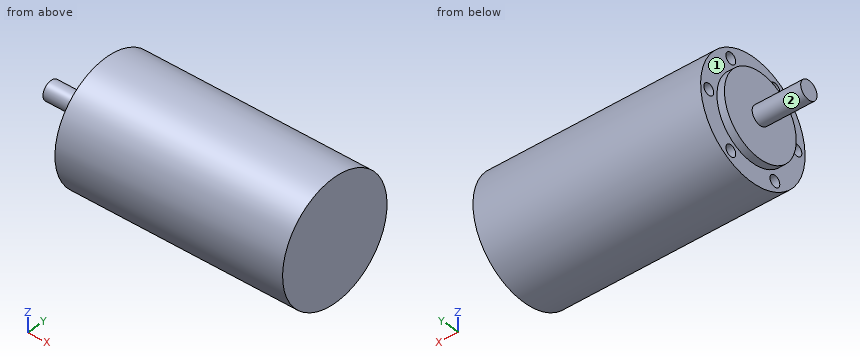
from build123d import *

# Parameters (mm, degrees)
SKETCH1_R           = 16
BOSS_EXTRUDE1_DEPTH = 61
SKETCH2_R           = 11
BOSS_EXTRUDE2_DEPTH = 2
SKETCH3_R           = 1.5
CUT_EXTRUDE1_DEPTH  = 4
SKETCH4_R           = 2.5
BOSS_EXTRUDE3_DEPTH = 13


with BuildPart() as part:
    # Sketch1 → Boss-Extrude1 (new body)
    with BuildSketch(Plane(origin=(0, 0, 0), x_dir=(0, 0, -1), z_dir=(1, 0, 0))):
        with Locations(Location((0, 0, 0), (0, 0, 180))):
            Circle(SKETCH1_R)
    extrude(amount=BOSS_EXTRUDE1_DEPTH)

    # Sketch2 → Boss-Extrude2 (add)
    with BuildSketch(Plane.ZY):
        Circle(SKETCH2_R)
    extrude(amount=BOSS_EXTRUDE2_DEPTH)

    # Sketch3 → Cut-Extrude1 (cut)
    with BuildSketch(Plane.ZY):
        with Locations((0, 13.5)):
            Circle(SKETCH3_R)
        with Locations((11.691342951, 6.75)):
            Circle(SKETCH3_R)
        with Locations((11.691342951, -6.75)):
            Circle(SKETCH3_R)
        with Locations((0, -13.5)):
            Circle(SKETCH3_R)
        with Locations((-11.691342951, -6.75)):
            Circle(SKETCH3_R)
        with Locations((-11.691342951, 6.75)):
            Circle(SKETCH3_R)
    extrude(amount=-CUT_EXTRUDE1_DEPTH, mode=Mode.SUBTRACT)

    # Sketch4 → Boss-Extrude3 (add)
    with BuildSketch(Plane.ZY.offset(2)):
        with Locations(Location((0, 0, 0), (0, 0, 180))):
            Circle(SKETCH4_R)
    extrude(amount=BOSS_EXTRUDE3_DEPTH)


solid = part.part
For this review, take the finished solid that the model builds, in its own axes (mm). Face numbers are marked on the shaded views. Round coordinates to 2 decimals unless told otherwise and drop trailing zeros. Loops run counter-clockwise (first coordinate to the right, second up) from the corner with the lowest first, then second, coordinate; pieces in that order, holes last. Notation, with made-up numbers: (30.5, 12.5) - (69.5, 12.5) arc R26 ccw to (69.5, 32.5) - close; hole circle Ø1 at (66, -38). An arc over 180 degrees is marked (long way). Answer as CSV lines item,"result".
(1) Consider section B-B on z = 0.5. Give the boundary of the cut face in (x, y), then the cut area to 3 significant figures.
Checked values:
outline,"(-15, -2.45) - (-2, -2.45) - (-2, -10.99) - (0, -10.99) - (0, -12.09) - (4, -12.09) - (4, -14.91) - (0, -14.91) - (0, -15.99) - (61, -15.99) - (61, 15.99) - (0, 15.99) - (0, 14.91) - (4, 14.91) - (4, 12.09) - (0, 12.09) - (0, 10.99) - (-2, 10.99) - (-2, 2.45) - (-15, 2.45) - close"
area,"2,040 mm2"
(2) Mouldability with a two-part tool opening along Y and no side actions: class the marked faces 1 and 2 as +Y half, -Y half, draft (parallel to the pull), parting line (faces both ways), or undercut.
Checked values:
face 1,"draft"
face 2,"parting line"
(3) Wall thickness on line 1 (Y direction, x = 3.5, z = -12); line 2 (X direction, y = 9.5, z = 8.5); line 3 (X direction, y = -5, z = 7.5): over which ranges is each line inside the solid? List them lowest first.
Checked values:
line 1,"y = -10.58 to -8.22, -5.28 to 5.28, 8.22 to 10.58"
line 2,"x = 0 to 61"
line 3,"x = -2 to 61"
(4) Consider section C-C on x = 36. Give the boundary of the cut face in (y, z).
Checked values:
outline,"circle Ø32 at (0, 0)"
(5) Consider section A-A on y = 0. Give the boundary of the cut face in (x, z), then the cut area to 3 significant figures.
Checked values:
outline,"(-15, -2.5) - (-2, -2.5) - (-2, -11) - (0, -11) - (0, -16) - (61, -16) - (61, 16) - (0, 16) - (0, 11) - (-2, 11) - (-2, 2.5) - (-15, 2.5) - close"
area,"2,060 mm2"
(6) Insertion check: P1, Ø5, axis at x = 42.5, y = 5.5, coming from the -Z side; P2, Ø4, axis at x = 46, z = -11.5, coming from the -Y side; P3, Ø0.9, axis at y = 6.5, z = 12, coming from the -X side. Each pin has a flat end and moves straight along its axis. Give the tip position at first contact, or say it passes through.
Checked values:
P1,"stops at z = -15.72"
P2,"stops at y = -12.87"
P3,"stops at x = 4"
(7) Consider section D-D on y = 6.75. Give the boundary of the cut face in (x, z).
Checked values:
outline,"(-2, -8.69) - (0, -8.69) - (0, -10.19) - (4, -10.19) - (4, -13.19) - (0, -13.19) - (0, -14.51) - (61, -14.51) - (61, 14.51) - (0, 14.51) - (0, 13.19) - (4, 13.19) - (4, 10.19) - (0, 10.19) - (0, 8.69) - (-2, 8.69) - close"
